from build123d import *

# Parameters (mm, degrees)
SKETCH1_W           = 110
SKETCH1_H           = 4
SKETCH1_W_2         = 4
SKETCH1_H_2         = 16
BOSS_EXTRUDE1_DEPTH = 20
SKETCH2_R           = 1.5
CUT_EXTRUDE1_DEPTH  = 114.243101335
SKETCH3_R           = 1.5
CUT_EXTRUDE2_DEPTH  = 62.846584384


with BuildPart() as part:
    # Sketch1 → Boss-Extrude1 (new body)
    with BuildSketch(Plane(origin=(0, 0, 0), x_dir=(1, 0, 0), z_dir=(0, 1, 0))):
        Rectangle(SKETCH1_W, SKETCH1_H)
        with Locations((-53, 10)):
            Rectangle(SKETCH1_W_2, SKETCH1_H_2)
        with Locations((53, 10)):
            Rectangle(SKETCH1_W_2, SKETCH1_H_2)
    extrude(amount=BOSS_EXTRUDE1_DEPTH)

    # Sketch2 → Cut-Extrude1 (cut, through all)
    with BuildSketch(Plane(origin=(55, 0, 0), x_dir=(0, 0, -1), z_dir=(1, 0, 0))):
        with Locations((12.593610515, 13.86730529)):
            Circle(SKETCH2_R)
        with Locations((13.103987848, 5.882981905)):
            Circle(SKETCH2_R)
    extrude(amount=-CUT_EXTRUDE1_DEPTH, mode=Mode.SUBTRACT)

    # Sketch3 → Cut-Extrude2 (cut, through all)
    with BuildSketch(Plane.XY.offset(2)):
        with Locations((22.5, 10)):
            Circle(SKETCH3_R)
        with Locations((-22.5, 10)):
            Circle(SKETCH3_R)
    extrude(amount=-CUT_EXTRUDE2_DEPTH, mode=Mode.SUBTRACT)


solid = part.part
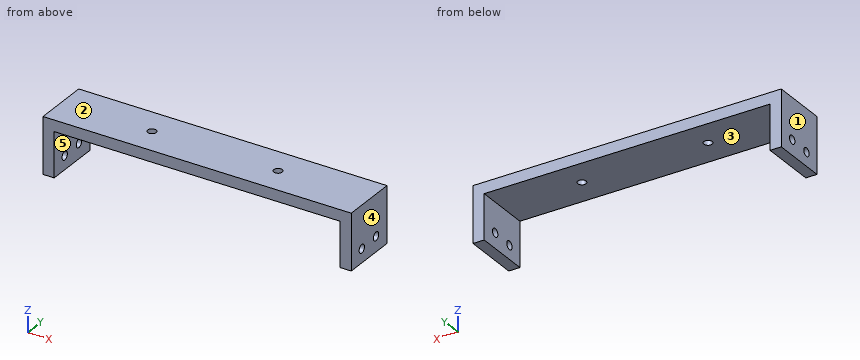
Part model, mm, in its own coordinate system. Face numbers are marked on the shaded views. A direction names the side the tool comes from. Round coordinates to 2 decimals unless told otherwise and drop trailing zeros. Write each loop counter-clockwise with the first axis right and the second up, starting at its lowest first coordinate (ties: lowest second). Pieces come first, ordered by that corner, then holes. Notation, with made-up numbers: M -20,80.25 L 18,80.25 A18 ccw 18,106.25 Z; hole C -40,41.25 d4. An arc over 180 degrees is marked long. Return JSON: item names as keys, results as strings. Group by question number.
(1) Pin check, flat tips, straight feed: pin 1 Ø4 at (x, y) = (22.5, 10) entering from -Z; pin 2 Ø2.5 at (y, z) = (5.88, -13.1) entering from -X. Stop position of each tip, or through.
(2) Saw through at C-C on y = 1.75. Write the cut outline in (x, z), then the cut area to 3 significant figures.
(3) Saw through at A-A on y = 10. Write the cut outline in (x, z).
(4) Saw through at B-B on x = 22.5. Write the cut outline in (y, z), then the cut area to 3 significant figures.
(5) Two-plate mould, pull along X, no slides. Class the marked faces 1, 2 and 3: +X half, -X half, draft (parallel to the pull), parting line (faces both ways), or undercut.
(6) Drill centre lines: probe 1 along X at (y, z) = (7, -3); probe 2 along Z at (x, y) = (30, 17.75); probe 3 along Y at (x, z) = (-22.5, -0.15). Where is each one in solid material? Low to high.
(7) Which spindle directions (+Z, -Z, +X, -X, +Y, -Y) get a long thin tool onto all of the face, cutting with end or side? Do the marked faces 4 and 5. Say none if no direction does.
Returned:
{
 "1": {"pin 1": "z = -2", "pin 2": "through"},
 "2": {"outline": "M -55,-18 L -51,-18 L -51,-2 L 51,-2 L 51,-18 L 55,-18 L 55,2 L -55,2 Z", "area": "568 mm²"},
 "3": {"outline": "M -55,-18 L -51,-18 L -51,-2 L -24,-2 L -24,2 L -55,2 Z; M -21,-2 L 21,-2 L 21,2 L -21,2 Z; M 24,-2 L 51,-2 L 51,-18 L 55,-18 L 55,2 L 24,2 Z"},
 "4": {"outline": "M 0,-2 L 8.5,-2 L 8.5,2 L 0,2 Z; M 11.5,-2 L 20,-2 L 20,2 L 11.5,2 Z", "area": "68.0 mm²"},
 "5": {"face 1": "-X half", "face 2": "draft", "face 3": "undercut"},
 "6": {"probe 1": "-55 to -51, 51 to 55", "probe 2": "-2 to 2", "probe 3": "0 to 8.5, 11.5 to 20"},
 "7": {"face 4": "+Z, -Z, +X, +Y, -Y", "face 5": "-Z, +Y, -Y"}
}
